from build123d import *

# Parameters (mm, degrees)
F1_DEPTH = 30


with BuildPart() as f1:
    # F0 (on Top) → F1 (new body)
    with BuildSketch(Plane.XY):
        with BuildLine():
            ThreePointArc((-13.5, 0), (-9.545942, 9.545942), (0, 13.5))
            Line((0, 13.5), (-13.5, 13.5))
            Line((-13.5, 13.5), (-18.5, 13.5))
            Line((-18.5, 13.5), (-18.5, 11.5))
            Line((-18.5, 11.5), (-13.5, 11.5))
            Line((-13.5, 11.5), (-13.5, 0))
        make_face()
        with BuildLine():
            Line((13.5, 0), (13.5, 11.5))
            Line((13.5, 11.5), (18.5, 11.5))
            Line((18.5, 11.5), (18.5, 13.5))
            Line((18.5, 13.5), (13.5, 13.5))
            Line((13.5, 13.5), (0, 13.5))
            ThreePointArc((0, 13.5), (9.545942, 9.545942), (13.5, 0))
        make_face()
        with BuildLine():
            ThreePointArc((7.5, -11.224972), (11.905881, -6.363961), (13.5, 0))
            ThreePointArc((13.5, 0), (9.545942, 9.545942), (0, 13.5))
            ThreePointArc((0, 13.5), (-9.545942, 9.545942), (-13.5, 0))
            ThreePointArc((-13.5, 0), (-11.905881, -6.363961), (-7.5, -11.224972))
            Line((-7.5, -11.224972), (-7.5, -7.348469))
            ThreePointArc((-7.5, -7.348469), (-3.968627, 9.721111), (10.5, 0))
            ThreePointArc((10.5, 0), (9.721111, -3.968627), (7.5, -7.348469))
            Line((7.5, -7.348469), (7.5, -11.224972))
        make_face()
    extrude(amount=F1_DEPTH)

    # F2 (on Front) → F3 (revolve, cut)
    with BuildSketch(Plane.XZ):
        Polygon((0, 0), (10.5, 0), (12.5, 30), (0, 30), align=None)
    revolve(axis=Axis((0, 0, 15), (0, 0, 1)), mode=Mode.SUBTRACT)


solid = f1.part
Geometry check sheet. Reference: the model listing, model coordinates, mm. A direction names the side the tool comes from. Round coordinates to 2 decimals unless told otherwise and drop trailing zeros. Loops run counter-clockwise (first coordinate to the right, second up) from the corner with the lowest first, then second, coordinate; pieces in that order, holes last. Notation, with made-up numbers: (66.25, 87) - (106.25, 87) arc R18 ccw to (106.25, 107) - close; hole circle Ø8 at (-9.75, 42.25). An arc over 180 degrees is marked (long way). One line per question, with ' | ' between items. Start each with the question number.
1. Draft check along X on faces 4 (the face through (-13.5, 6, 15)), 5 (the face through (-16, 11.5, 15)), 6 (the face through (7.5, -10, 11)), 7 (the face through (18.5, 12, 15)). Enter one of: released by +X, released by -X, zero draft, split by the parting line, or undercut.
2. Tool access check on faces 1 (the face through (-18.5, 13, 15)), 2 (the face through (13.5, 6, 15)), 3 (the face through (-7.5, -10, 11)). Record the directions out of +Z, -Z, +X, -X, +Y, -Y that give a thin tool (end or side, any length) a straight path to the whole face; none if there is none.
3. Depth check by flat-ended pin: pin 1 (3.5 mm diameter, centred on y = 4.5, z = 21.5, fed in from -X); pin 2 (6 mm diameter, centred on y = 3.5, z = 16, fed in from +X); pin 3 (1.9 mm diameter, centred on y = -10, z = 21.5, fed in from -X). Enter the tip coordinate at first touch or a pass-through.
4. Cross-section at C-C on z = 14.25. Record the cut outline in (x, y).
5. Cross-section at A-A on z = 3.75. Record the cut outline in (x, y), then the cut area to 3 significant figures.
6. Cross-section at B-B on x = 0. Record the cut outline in (y, z).
7. Scan lines: line 1 (X direction, y = 4.5, z = 9.5); line 2 (X direction, y = -5.5, z = 21.75); line 3 (Y direction, x = -14, z = 8.5). Record each from-to range of solid material in increasing order. Write a range as [from, to].
Taken from the geometry:
1) face 4: released by -X | face 5: zero draft | face 6: undercut | face 7: released by +X
2) face 1: +Z, -Z, -X, +Y, -Y | face 2: +Z, -Z, +X, -Y | face 3: +Z, -Z, -Y
3) pin 1: x = -13.5 | pin 2: x = 13.5 | pin 3: x = -10.02
4) outline: (-18.5, 11.5) - (-13.5, 11.5) - (-13.5, 0) arc R13.5 ccw to (-7.5, -11.22) - (-7.5, -8.65) arc R11.45 cw (long way) to (7.5, -8.65) - (7.5, -11.22) arc R13.5 ccw to (13.5, 0) - (13.5, 11.5) - (18.5, 11.5) - (18.5, 13.5) - (-18.5, 13.5) - close
5) outline: (-18.5, 11.5) - (-13.5, 11.5) - (-13.5, 0) arc R13.5 ccw to (-7.5, -11.22) - (-7.5, -7.7) arc R10.75 cw (long way) to (7.5, -7.7) - (7.5, -11.22) arc R13.5 ccw to (13.5, 0) - (13.5, 11.5) - (18.5, 11.5) - (18.5, 13.5) - (-18.5, 13.5) - close | area: 263 mm²
6) outline: (10.5, 0) - (13.5, 0) - (13.5, 30) - (12.5, 30) - close
7) line 1: [-13.5, -10.18], [10.18, 13.5] | line 2: [-12.33, -10.61], [10.61, 12.33] | line 3: [11.5, 13.5]
